from build123d import *
from build123d.topology import SkipClean

# Parameters (mm, degrees)
SKETCH_1_R               = 2.35
SKETCH_1_R_2             = 1.3
EXTRUDE_1_DEPTH          = 2.5
EXTRUDE_1_2_DEPTH        = 2.5
EXTRUDE_1_3_DEPTH        = 2.5
EXTRUDE_1_4_DEPTH        = 2.5
SKETCH_2_R               = 17.75
EXTRUDE_2_DEPTH          = 2
SKETCH_3_R               = 1.3
CUT_EXTRUDE_1_DEPTH      = 26.226474189
CUT_EXTRUDE_2_DEPTH      = 26.502450863
CUT_EXTRUDE_2_DEPTH_BACK = 26.502450863
EXTRUDE_START            = 7.5
SKETCH_5_R               = 17.75
SKETCH_5_R_2             = 17.15
EXTRUDE_3_DEPTH          = 7.5
SKETCH_6_W               = 4
SKETCH_6_H               = 5
CUT_EXTRUDE_3_DEPTH      = 4.5
CUT_EXTRUDE_4_DEPTH      = 27.839802533
CUT_EXTRUDE_5_DEPTH      = 3.5
FILLET_1_R               = 2


with BuildPart() as part:
    # Sketch 1 → Extrude 1 (new body)
    with BuildSketch(Plane(origin=(0, 0, 0), x_dir=(1, 0, 0), z_dir=(0, 1, 0))):
        with Locations(Location((0, 8, 0), (0, 0, 270))):
            Circle(SKETCH_1_R)
        with Locations(Location((0, 8, 0), (0, 0, 270))):
            Circle(SKETCH_1_R_2, mode=Mode.SUBTRACT)
    extrude(amount=EXTRUDE_1_DEPTH)



with BuildPart() as body_2:
    # Sketch 1 → Extrude 1 2 (new body)
    with BuildSketch(Plane(origin=(0, 0, 0), x_dir=(1, 0, 0), z_dir=(0, 1, 0))):
        with Locations(Location((8, 0, 0), (0, 0, 270))):
            Circle(SKETCH_1_R)
        with Locations(Location((8, 0, 0), (0, 0, 270))):
            Circle(SKETCH_1_R_2, mode=Mode.SUBTRACT)
    extrude(amount=EXTRUDE_1_2_DEPTH)


with BuildPart() as body_3:
    # Sketch 1 → Extrude 1 3 (new body)
    with BuildSketch(Plane(origin=(0, 0, 0), x_dir=(1, 0, 0), z_dir=(0, 1, 0))):
        with Locations(Location((0, -8, 0), (0, 0, 270))):
            Circle(SKETCH_1_R)
        with Locations(Location((0, -8, 0), (0, 0, 270))):
            Circle(SKETCH_1_R_2, mode=Mode.SUBTRACT)
    extrude(amount=EXTRUDE_1_3_DEPTH)


with BuildPart() as body_4:
    # Sketch 1 → Extrude 1 4 (new body)
    with BuildSketch(Plane(origin=(0, 0, 0), x_dir=(1, 0, 0), z_dir=(0, 1, 0))):
        with Locations(Location((-8, 0, 0), (0, 0, 270))):
            Circle(SKETCH_1_R)
        with Locations(Location((-8, 0, 0), (0, 0, 270))):
            Circle(SKETCH_1_R_2, mode=Mode.SUBTRACT)
    extrude(amount=EXTRUDE_1_4_DEPTH)


with BuildPart() as part_1:
    add(part.part)

    add(body_2.part)  # Extrude 2 merges body 2

    add(body_3.part)  # Extrude 2 merges body 3

    add(body_4.part)  # Extrude 2 merges body 4
    # Sketch 2 → Extrude 2 (add)
    with BuildSketch(Plane(origin=(0, 2.5, 0), x_dir=(1, 0, 0), z_dir=(0, 1, 0))):
        with Locations(Location((0, 0, 0), (0, 0, 270))):
            Circle(SKETCH_2_R)
    extrude(amount=EXTRUDE_2_DEPTH)

    # Sketch 3 → Cut-Extrude 1 (cut, through all)
    with BuildSketch(Plane.XZ.offset(-2.5)):
        with Locations(Location((0, -8, 0), (0, 0, 270))):
            Circle(SKETCH_3_R)
        with Locations(Location((8, 0, 0), (0, 0, 270))):
            Circle(SKETCH_3_R)
        with Locations(Location((0, 8, 0), (0, 0, 270))):
            Circle(SKETCH_3_R)
        with Locations(Location((-8, 0, 0), (0, 0, 270))):
            Circle(SKETCH_3_R)
    extrude(amount=-CUT_EXTRUDE_1_DEPTH, mode=Mode.SUBTRACT)

    # Sketch 4 → Cut-Extrude 2 (cut, two sides: drawn at the far end of the back side and taken through both)
    with BuildSketch(Plane(origin=(0, 4.5, 0), x_dir=(1, 0, 0), z_dir=(0, 1, 0)).offset(-CUT_EXTRUDE_2_DEPTH_BACK)):
        Polygon((8.067949046, 9.464101393), (12.067949458, 2.535898401), (15.532050954, 4.535898607), (11.532050542, 11.464101599), align=None)
    extrude(amount=CUT_EXTRUDE_2_DEPTH + CUT_EXTRUDE_2_DEPTH_BACK, mode=Mode.SUBTRACT)

    # Sketch 5 → Extrude 3 (add)
    with BuildSketch(Plane.XZ.offset(-2.5).offset(EXTRUDE_START)):
        with Locations(Location((0, 0, 0), (0, 0, 270))):
            Circle(SKETCH_5_R)
        with Locations(Location((0, 0, 0), (0, 0, 270))):
            Circle(SKETCH_5_R_2, mode=Mode.SUBTRACT)
    extrude(amount=-EXTRUDE_3_DEPTH)

    # Sketch 6 → Cut-Extrude 3 (cut)
    with BuildSketch(Plane(origin=(0, 4.5, 0), x_dir=(1, 0, 0), z_dir=(0, 1, 0))):
        with Locations((15.75, 0)):
            Rectangle(SKETCH_6_W, SKETCH_6_H)
    extrude(amount=-CUT_EXTRUDE_3_DEPTH, mode=Mode.SUBTRACT)

    # Sketch 7 → Cut-Extrude 4 (cut, through all)
    with SkipClean():  # the faces are left unmerged after this step: merging them gives an invalid solid
        with BuildSketch(Plane(origin=(0, 4.5, 0), x_dir=(1, 0, 0), z_dir=(0, 1, 0))):
            with BuildLine():
                Line((11.409480072, -13.597288865), (7.874148219, -9.384044428))
                ThreePointArc((7.874148219, -9.384044428), (1.386739369, -12.171255232), (-5.561383622, -10.914829921))
                Line((-5.561383622, -10.914829921), (-8.05833137, -15.815365804))
                ThreePointArc((-8.05833137, -15.815365804), (2.009357044, -17.635900438), (11.409480072, -13.597288865))
            make_face()
        extrude(amount=-CUT_EXTRUDE_4_DEPTH, mode=Mode.SUBTRACT)

    # Sketch 8 → Cut-Extrude 5 (cut)
    with SkipClean():  # the faces are left unmerged after this step: merging them gives an invalid solid
        with BuildSketch(Plane.XZ.offset(5)):
            with BuildLine():
                Line((-4.594038051, -17.145183417), (-4.438746624, -16.565627921))
                ThreePointArc((-4.438746624, -16.565627921), (0, -17.15), (4.438746624, -16.565627921))
                Line((4.438746624, -16.565627921), (4.594038051, -17.145183417))
                ThreePointArc((4.594038051, -17.145183417), (0, -17.75), (-4.594038051, -17.145183417))
            make_face()
        extrude(amount=-CUT_EXTRUDE_5_DEPTH, mode=Mode.SUBTRACT)

    # Fillet 1
    # the kernel refuses this fillet: 2 mm, written as the material it adds along each edge
    with BuildSketch(Plane(origin=(-5.561383622, 4.5, 10.914829921), x_dir=(-0.4539904997395411, 0, 0.8910065241883708), z_dir=(0, -1, 0))) as fillet_1_piece_1:
        with BuildLine():
            CenterArc((1.85895106, -2), FILLET_1_R, 90, 81.9318495)
            ThreePointArc((-0.121252598, -1.719298246), (-0.030350748, -0.86178429), (0, 0))
            Line((0, 0), (1.85895106, 0))
        make_face()
    extrude(amount=2)
    with BuildSketch(Plane(origin=(7.874148219, 4.5, 9.384044428), x_dir=(-0.8093664220446892, 0, 0.5873040054916857), z_dir=(0, -1, 0))) as fillet_1_piece_2:
        with BuildLine():
            CenterArc((1.864268056, -1.995044776), FILLET_1_R, 94.03407525, 81.9318495)
            Line((-0.13077672, -1.8543453), (0, 0))
            ThreePointArc((0, 0), (0.86178429, -0.030350748), (1.72356858, 0))
        make_face()
    extrude(amount=2)
    # the kernel refuses this fillet: 2 mm, written as the material it takes off along each edge
    with BuildSketch(Plane(origin=(-8.05833137, 2.5, 15.815365804), x_dir=(0.45399049973954037, 0, -0.8910065241883711), z_dir=(0, -1, 0))) as fillet_1_2_piece_1:
        with BuildLine():
            CenterArc((2.1275002, -2), FILLET_1_R, 90, 97.295351085)
            ThreePointArc((0.143690702, -2.253968254), (0.0359591, -1.129271879), (0, 0))
            Line((0, 0), (2.1275002, 0))
        make_face()
    extrude(amount=13.146359395, mode=Mode.SUBTRACT)
    with BuildSketch(Plane(origin=(11.409480072, 2.5, 13.597288865), x_dir=(0.7235977816974914, 0, -0.6902218848475246), z_dir=(0, -1, 0))) as fillet_1_2_piece_2:
        with BuildLine():
            CenterArc((2.131301856, -1.99594827), FILLET_1_R, 86.352324458, 97.295351085)
            Line((0.135353586, -2.123190172), (0, 0))
            ThreePointArc((0, 0), (1.129271879, 0.0359591), (2.258543758, 0))
        make_face()
    extrude(amount=13.146359395, mode=Mode.SUBTRACT)
    with BuildSketch(Plane(origin=(11.409480072, 10.146359395, 13.597288865), x_dir=(0.7235977816974903, 0, -0.6902218848475259), z_dir=(0, -1, 0))) as fillet_1_2_piece_3:
        with BuildLine():
            CenterArc((2.131301856, -1.99594827), FILLET_1_R, 86.352324458, 97.295351085)
            Line((0.135353586, -2.123190172), (0, 0))
            ThreePointArc((0, 0), (1.129271879, 0.0359591), (2.258543758, 0))
        make_face()
    extrude(amount=7.646359395, mode=Mode.SUBTRACT)
    with BuildSketch(Plane(origin=(-8.05833137, 10.146359395, 15.815365804), x_dir=(-0.8603181581586984, 0, -0.5097574587413362), z_dir=(0, -1, 0))) as fillet_1_2_piece_4:
        with BuildLine():
            CenterArc((2.131301856, 1.99594827), FILLET_1_R, 176.352324458, 97.295351085)
            Line((0.135353586, 2.123190172), (0, 0))
            ThreePointArc((0, 0), (1.129271879, -0.0359591), (2.258543758, 0))
        make_face()
    extrude(amount=7.646359395, mode=Mode.SUBTRACT)


solid = part_1.part
Source: CAD feature listing. Evaluate the final solid. Frame: model axes, mm. A direction names the side the tool comes from. Round coordinates to 2 decimals unless told otherwise and drop trailing zeros. Write each loop counter-clockwise with the first axis right and the second up, starting at its lowest first coordinate (ties: lowest second). Pieces come first, ordered by that corner, then holes. Notation, with made-up numbers: M -40,16.25 L -6,16.25 A7 ccw -6,24.25 Z; hole C 40,5 d8. An arc over 180 degrees is marked long. One line per item, written item: value. Start each with the question number.
Item 1: Section query D-D (y = 3). Return the cut outline in (x, z), plus the area to 3 significant figures.
Item 2: Pin query (flat end, axial travel): pin 1 (3.5 mm diameter, centred on x = 0, z = 8, fed in from -Y); pin 2 (3 mm diameter, centred on x = -5, y = -1, fed in from -Z); pin 3 (2 mm diameter, centred on y = -3, z = -8, fed in from +X); pin 4 (2.5 mm diameter, centred on x = -8, z = 0, fed in from -Y). Return the tip coordinate at first contact, or that it passes through.
Item 3: Mould query, pull axis X, two halves, no side actions, for faces 1 (the flat face through (13.75, 4, 0)), 2 (the flat face through (-17, -5, -3.4)), 3 (the flat face through (13.56, 3.49, -7.95)). Classes: pulls with the +X half, pulls with the -X half, needs draft (parallel to the pull), parting line crosses it, or undercut.
Item 4: Section query C-C (z = 8). Return the cut outline in (x, y), plus the area to 3 significant figures.
Item 5: Ray query, L1, parallel to X at y = 3.5, z = 0; L2, parallel to X at y = 0.8, z = 0; L3, parallel to X at y = 2.25, z = 1. Return the intervals inside material, ascending. Write a range as from..to.
Item 6: Section query A-A (z = 0). Return the cut outline in (x, y).
Item 7: Set-up query: faces 4 (the cylindrical face through (-10.294, 1.232, -0.509)), 5 (the flat face through (13.776, 3.486, -3.522)), 6 (the cylindrical face through (7.831, 3.514, 10.115)), 7 (the flat face through (-2, 0, 8)). Return all of +Z, -Z, +X, -X, +Y, -Y with unobstructed straight access to the full face (end or side cutting, diameter ignored); none if empty.
Item 8: Section query B-B (x = -8). Return the cut outline in (y, z).
Result set:
1. outline: M -10,14.66 A17.75 ccw long 17.57,-2.5 L 13.75,-2.5 L 13.75,2.5 L 17.57,2.5 A17.75 ccw 13.04,12.04 A2 ccw 10.04,11.97 L 9.07,10.81 A2 cw 6.48,10.4 A12.25 ccw -3.97,11.59 A2 cw -6.41,12.57 L -7.09,13.92 A2 ccw Z; hole C -8,0 d2.6; hole C 0,-8 d2.6; hole C 0,8 d2.6; hole C 8,0 d2.6; hole M 8.07,-9.46 L 11.53,-11.46 L 15.53,-4.54 L 12.07,-2.54 Z
1. area: 820 mm²
2. pin 1: stops at y = 0
2. pin 2: stops at z = -17.4
2. pin 3: stops at x = 16.31
2. pin 4: passes through
3. face 1: pulls with the +X half
3. face 2: needs draft
3. face 3: undercut
4. outline: M -15.84,-5 L -15.17,-5 L -15.17,2.5 L -2.35,2.5 L -2.35,0 L -1.3,0 L -1.3,4.5 L -15.84,4.5 Z; M 1.3,0 L 2.35,0 L 2.35,2.5 L 15.17,2.5 L 15.17,-5 L 15.84,-5 L 15.84,4.5 L 1.3,4.5 Z
4. area: 73.6 mm²
5. L1: x = -17.75..-9.3, -6.7..6.7, 9.3..13.75
5. L2: x = -17.75..-17.15, -10.35..-9.3, -6.7..-5.65, 5.65..6.7, 9.3..10.35
5. L3: x = -17.72..-17.12, -10.13..-8.83, -7.17..-5.87, 5.87..7.17, 8.83..10.13
6. outline: M -17.75,-5 L -17.15,-5 L -17.15,2.5 L -10.35,2.5 L -10.35,0 L -9.3,0 L -9.3,4.5 L -17.75,4.5 Z; M -6.7,0 L -5.65,0 L -5.65,2.5 L 5.65,2.5 L 5.65,0 L 6.7,0 L 6.7,4.5 L -6.7,4.5 Z; M 9.3,0 L 10.35,0 L 10.35,2.5 L 13.75,2.5 L 13.75,4.5 L 9.3,4.5 Z; M 17.15,-5 L 17.75,-5 L 17.75,0 L 17.15,0 Z
7. face 4: -Y
7. face 5: +Y, -Y
7. face 6: +Z, +Y, -Y
7. face 7: +Z, -Y
8. outline: M -5,-15.84 L 4.5,-15.84 L 4.5,-1.3 L 0,-1.3 L 0,-2.35 L 2.5,-2.35 L 2.5,-15.17 L -5,-15.17 Z; M 0,1.3 L 4.5,1.3 L 4.5,14.81 L 2.5,14.81 L 2.5,2.35 L 0,2.35 Z
